Check sheet for the modelled part. Datum: model origin and axes. Units: mm. Round coordinates to 2 decimals unless told otherwise and drop trailing zeros. Write each loop counter-clockwise with the first axis right and the second up, starting at its lowest first coordinate (ties: lowest second). Pieces come first, ordered by that corner, then holes.
Item 1: Material ranges on line 1 (X direction, y = -11, z = -26); line 2 (Z direction, x = 35.5, y = -8.5); line 3 (Z direction, x = -21, y = -10), recorded low to high.
Item 2: Go/stop test with flat-tipped pins: pin 1 Ø2 at (y, z) = (-2.5, -15.5) entering from +X; pin 2 Ø1 at (y, z) = (-7, -12.5) entering from +X; pin 3 Ø1.5 at (x, y) = (-23, -5.5) entering from -Z. Record where each tip stops, or that it passes through.
Item 3: Cross-section at C-C on x = 12.5. Enter the section's corners in (y, z).
Item 4: Cross-section at B-B on z = -16. Enter the section's corners in (x, y).
Item 5: Cross-section at A-A on y = -4.5. Enter the section's corners in (x, z) (3 decimals), plus the area to 3 significant figures.
from build123d import *

# Parameters (mm, degrees)
F1_DEPTH = 12.7


with BuildPart() as f1:
    # F0 (on Front) → F1 (new body)
    with BuildSketch(Plane.XZ):
        with BuildLine():
            Line((32.995568, 25.4), (-32.995568, 25.4))
            ThreePointArc((-32.995568, 25.4), (-38.494829, 22.225), (-38.494829, 15.875))
            Line((-38.494829, 15.875), (-5.499261, -41.275))
            ThreePointArc((-5.499261, -41.275), (0, -44.45), (5.499261, -41.275))
            Line((5.499261, -41.275), (38.494829, 15.875))
            ThreePointArc((38.494829, 15.875), (38.494829, 22.225), (32.995568, 25.4))
        make_face()
    extrude(amount=F1_DEPTH)


solid = f1.part
Response values:
1. line 1: x = -14.32 to 14.32
1. line 2: z = 10.69 to 24.89
1. line 3: z = -14.43 to 25.4
2. pin 1: stops at x = 20.96
2. pin 2: stops at x = 22.4
2. pin 3: stops at z = -12.26
3. outline: (-12.7, -29.15) - (0, -29.15) - (0, 25.4) - (-12.7, 25.4) - close
4. outline: (-20.09, -12.7) - (20.09, -12.7) - (20.09, 0) - (-20.09, 0) - close
5. outline: (-38.495, 15.875) - (-5.499, -41.275) arc R6.35 ccw to (5.499, -41.275) - (38.495, 15.875) arc R6.35 ccw to (32.996, 25.4) - (-32.996, 25.4) arc R6.35 ccw to start
5. area: 3,270 mm2
